Can you work these out from the drawing? Everything is in mm from the part's minimum corner. A direction names the side the tool comes from. Round coordinates to 2 decimals unless told otherwise and drop trailing zeros. Write each loop counter-clockwise with the first axis right and the second up, starting at its lowest first coordinate (ties: lowest second). Pieces come first, ordered by that corner, then holes. Notation, with made-up numbers: (57.5, 38.25) -> (62.5, 38.25) arc R23 cw to (62.5, 77.25) -> close; hole circle Ø6 at (78, 4). An arc over 180 degrees is marked (long way). Write item = value, one per line. Start each with the question number.
1) Imagine slicing it at B-B, the plane z = 30. Please give me the cut outline in (x, y).
2) I'm going to push flat-ended pins straight in: pin 1 (7.5 mm diameter, centred on x = 23.5, y = 17, fed in from +Z); pin 2 (5 mm diameter, centred on x = 60.5, y = 16.5, fed in from -Z); pin 3 (12.5 mm diameter, centred on y = 8, z = 29.5, fed in from -X). Where does each tip first touch, or does it pass through?
3) Imagine slicing it at C-C, the plane x = 16.5. Please give me the cut outline in (y, z).
4) If I drill on line 1 (X direction, y = 7, z = 44); line 2 (Z direction, x = 12, y = 20.75), over which ranges is the centre line in solid material (lowest first)?
5) For the marked faces 1 and 2, which set-ups out of +Z, -Z, +X, -X, +Y, -Y let a thin tool reach every point of the face, with its end or its side?
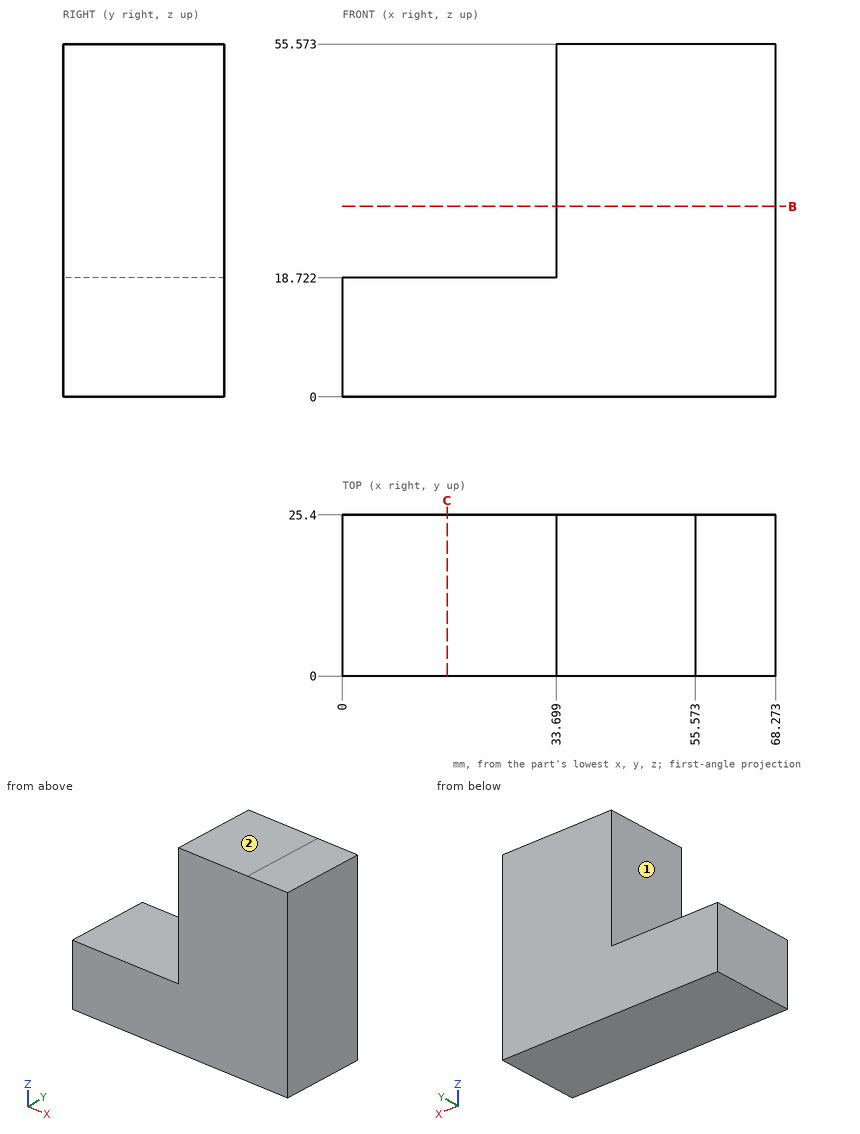
Reported:
q1.outline = (33.7, 0) -> (68.27, 0) -> (68.27, 25.4) -> (33.7, 25.4) -> close
q2.pin_1 = 18.72
q2.pin_2 = 0
q2.pin_3 = 33.7
q3.outline = (0, 0) -> (25.4, 0) -> (25.4, 18.72) -> (0, 18.72) -> close
q4.line_1 = 33.7 to 68.27
q4.line_2 = 0 to 18.72
q5.face_1 = +Z, -X, +Y, -Y
q5.face_2 = +Z, +X, -X, +Y, -Y
